Input: part model. Units: mm. Frame: model coordinates. Face numbers are marked on the shaded views. A direction names the side the tool comes from. Round coordinates to 2 decimals unless told otherwise and drop trailing zeros. Loops run counter-clockwise (first coordinate to the right, second up) from the corner with the lowest first, then second, coordinate; pieces in that order, holes last. Notation, with made-up numbers: (82.5, 62) -> (103.5, 62) arc R19 ccw to (103.5, 95) -> close; hole circle Ø4 at (46, -24.75). An arc over 180 degrees is marked (long way). Answer as a JSON object with one key per item and string values. Group by question number.
Item 1: Set-up query: the marked faces 4 and 5. Return all of +Z, -Z, +X, -X, +Y, -Y with unobstructed straight access to the full face (end or side cutting, diameter ignored); none if empty.
Item 2: Section query C-C on z = -0.5. Return loops of the section in (x, y), and give its area (3 significant figures).
Item 3: Material intervals for line 1 (Z direction, x = -3, y = -7.75); line 2 (Y direction, x = 5.75, z = 2.5); line 3 (X direction, y = -6, z = 1), sorted ascending. Write a range as [from, to].
Item 4: Section query A-A on z = -3.25. Return loops of the section in (x, y).
Item 5: Draft query along Y for the marked faces 1, 2 and 3. Return one class per face: released by +Y, released by -Y, zero draft, split by the parting line, or undercut.
Item 6: Pin query (flat end, axial travel): pin 1 (5.5 mm diameter, centred on x = -1, y = 1, fed in from -Z); pin 2 (8 mm diameter, centred on x = 7, y = -4.5, fed in from -Z). Return the tip coordinate at first contact, or that it passes through.
Item 7: Section query B-B on y = -8.5. Return loops of the section in (x, z), and give its area (3 significant figures).
from build123d import *

# Parameters (mm, degrees)
SKETCH1_R           = 4.0386
BOSS_EXTRUDE1_DEPTH = 2.54
SKETCH1_4_R         = 10.9855
SKETCH1_4_R_2       = 4.0386
BOSS_EXTRUDE2_DEPTH = 3.81
FILLET1_R           = 2.54
FILLET2_R           = 12.7
SKETCH1_6_R         = 4.0386
BOSS_EXTRUDE3_DEPTH = 6.35
SKETCH3_R           = 2.54
CUT_EXTRUDE1_DEPTH  = 3.81


with BuildPart() as part:
    # Sketch1 → Boss-Extrude1 (new body)
    with BuildSketch(Plane.XY):
        Circle(SKETCH1_R)
    extrude(amount=BOSS_EXTRUDE1_DEPTH)

    # Sketch1<4> → Boss-Extrude2 (add)
    with BuildSketch(Plane.XY):
        with Locations(Location((0, 0, 0), (0, 0, 180))):
            Circle(SKETCH1_4_R)
        with Locations(Location((0, 0, 0), (0, 0, 180))):
            Circle(SKETCH1_4_R_2, mode=Mode.SUBTRACT)
    extrude(amount=BOSS_EXTRUDE2_DEPTH)

    # Fillet1
    # the kernel refuses this fillet: 2.54 mm, written as the material it takes off along each edge
    with BuildSketch(Plane(origin=(0, 0, 3.81), x_dir=(-1, 0, 0), z_dir=(0, 1, 0))) as fillet1_piece_1:
        with BuildLine():
            CenterArc((6.238304526, -2.54), FILLET1_R, 90, 60)
            Line((4.0386, -1.27), (3.994605909, -1.2446))
            ThreePointArc((3.994605909, -1.2446), (3.9878, -0.635), (3.9878, 0))
            Line((3.9878, 0), (4.0386, 0.0508))
            Line((4.0386, 0.0508), (6.238304526, 0.0508))
            Line((6.238304526, 0.0508), (6.238304526, 0))
        make_face()
    revolve(axis=Axis((0, 0, 3.81), (0, 0, 1)), mode=Mode.SUBTRACT)

    # Fillet2
    fillet2_edges = [part.edges().sort_by_distance(p)[0] for p in [
        (4.0386, 0, 2.54),
    ]]
    fillet(fillet2_edges, radius=FILLET2_R)

    # Sketch1<6> → Boss-Extrude3 (add)
    with BuildSketch(Plane.XY):
        Circle(SKETCH1_6_R)
    extrude(amount=-BOSS_EXTRUDE3_DEPTH)

    # Sketch3 → Cut-Extrude1 (cut)
    with BuildSketch(Plane(origin=(0, 0, -6.35), x_dir=(-1, 0, 0), z_dir=(0, 0, -1))):
        Circle(SKETCH3_R)
    extrude(amount=-CUT_EXTRUDE1_DEPTH, mode=Mode.SUBTRACT)


solid = part.part
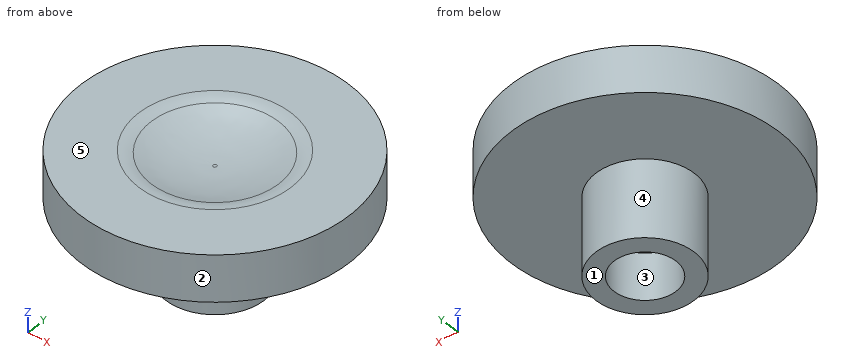
Solved:
{
 "1": {"face 4": "-Z", "face 5": "+Z, +X, -X, +Y, -Y"},
 "2": {"outline": "circle Ø8.08 at (0, 0)", "area": "51.2 mm²"},
 "3": {"line 1": "[0, 3.81]", "line 2": "[-9.36, 9.36]", "line 3": "[-9.2, 9.2]"},
 "4": {"outline": "circle Ø8.08 at (0, 0); hole circle Ø5.08 at (0, 0)"},
 "5": {"face 1": "zero draft", "face 2": "split by the parting line", "face 3": "undercut"},
 "6": {"pin 1": "z = -6.35", "pin 2": "z = 0"},
 "7": {"outline": "(-6.96, 0) -> (6.96, 0) -> (6.96, 3.81) -> (-6.96, 3.81) -> close", "area": "53.0 mm²"}
}
